Verification items for the finished model (mm, model axes). A direction names the side the tool comes from. Give positions to 0.01 mm unless a question says otherwise; leave off trailing zeros. Loops run counter-clockwise (first coordinate to the right, second up) from the corner with the lowest first, then second, coordinate; pieces in that order, holes last. Notation, with made-up numbers: (88.5, 40) - (102.5, 40) arc R26 cw to (102.5, 77) - close; hole circle Ø8 at (87, 27). An arc over 180 degrees is marked (long way). Answer in a Markdown table with one row per item.
```python
from build123d import *

# Parameters (mm, degrees)
F0_W     = 254
F0_H     = 76.2
F1_DEPTH = 6.35
F2_W     = 6.35
F2_H     = 6.35
F2_H_2   = 12.7
F2_H_3   = 31.75
F3_DEPTH = 6.35
F4_W     = 30.48
F4_H     = 6.35
F5_DEPTH = 6.351
F6_W     = 6.35
F6_H     = 12.7
F7_DEPTH = 6.351


with BuildPart() as f1:
    # F0 (on Front) → F1 (new body)
    with BuildSketch(Plane.XZ):
        with Locations((127, 38.1)):
            Rectangle(F0_W, F0_H)
    extrude(amount=F1_DEPTH)

    # F2 (on face) → F3 (cut, through all)
    with BuildSketch(Plane.XZ.offset(6.35)):
        with Locations((3.175, 3.175)):
            Rectangle(F2_W, F2_H)
        with Locations((3.175, 69.85)):
            Rectangle(F2_W, F2_H_2)
        with Locations((3.175, 34.925)):
            Rectangle(F2_W, F2_H_3)
        with Locations((250.825, 3.175)):
            Rectangle(F2_W, F2_H)
        with Locations((250.825, 34.925)):
            Rectangle(F2_W, F2_H_3)
        with Locations((250.825, 69.85)):
            Rectangle(F2_W, F2_H_2)
    extrude(amount=-F3_DEPTH, mode=Mode.SUBTRACT)

    # F4 (on face) → F5 (cut, through all)
    with BuildSketch(Plane.XZ.offset(6.35)):
        with Locations((15.24, 3.175)):
            Rectangle(F4_W, F4_H)
        with Locations((71.12, 3.175)):
            Rectangle(F4_W, F4_H)
        with Locations((127, 3.175)):
            Rectangle(F4_W, F4_H)
        with Locations((182.88, 3.175)):
            Rectangle(F4_W, F4_H)
        with Locations((238.76, 3.175)):
            Rectangle(F4_W, F4_H)
    extrude(amount=-F5_DEPTH, mode=Mode.SUBTRACT)

    # F6 (on face) → F7 (cut, through all)
    with BuildSketch(Plane.XZ.offset(6.35)):
        with Locations((85.725, 12.7)):
            Rectangle(F6_W, F6_H)
        with Locations((85.725, 57.15)):
            Rectangle(F6_W, F6_H)
        with Locations((168.275, 57.15)):
            Rectangle(F6_W, F6_H)
        with Locations((168.275, 12.7)):
            Rectangle(F6_W, F6_H)
    extrude(amount=-F7_DEPTH, mode=Mode.SUBTRACT)


solid = f1.part
```
Q1. Tool access check on faces 4 (the face through (251, -3, 63.5)), 5 (the face through (86, -3, 19.05)), 6 (the face through (239, -3, 6.35)), 7 (the face through (82.55, -3, 13)). Record the directions out of +Z, -Z, +X, -X, +Y, -Y that give a thin tool (end or side, any length) a straight path to the whole face; none if there is none.
Completed:
| item | result |
|---|---|
| face 4 | +Z, +X, +Y, -Y |
| face 5 | +Y, -Y |
| face 6 | -Z, +X, +Y, -Y |
| face 7 | -Z, +Y, -Y |
Q2. Draft check along X on faces 1 (the face through (168, -3, 50.8)), 2 (the face through (251, -3, 19.05)), 3 (the face through (254, -3, 57)). Enter one of: +X half, -X half, draft (parallel to the pull), parting line (faces both ways), or undercut.
Completed:
| item | result |
|---|---|
| face 1 | undercut |
| face 2 | draft |
| face 3 | +X half |
Q3. Sectioned sample at A-A (x = 135). Record the cut outline in (y, z), and give its area (3 significant figures).
Completed:
| item | result |
|---|---|
| outline | (-6.35, 6.35) - (0, 6.35) - (0, 76.2) - (-6.35, 76.2) - close |
| area | 444 mm^2 |
Q4. Sectioned sample at C-C (z = 40). Record the cut outline in (x, y).
Completed:
| item | result |
|---|---|
| outline | (6.35, -6.35) - (247.65, -6.35) - (247.65, 0) - (6.35, 0) - close |
Q5. Sectioned sample at B-B (y = -2.75). Give the number of separate pieces and of enclosed holes in the cut face, and give its area (3 significant figures).
Completed:
| item | result |
|---|---|
| separate pieces | 1 |
| enclosed holes | 2 |
| area | 17,500 mm^2 |
Q6. Go/stop test with flat-tipped pins: P1, Ø3, axis at x = 4, y = -2, coming from the -Z side; P2, Ø2, axis at y = -4.5, z = 22, coming from the -X side; P3, Ø1.9, axis at y = -2.5, z = 4.5, coming from the +X side. Record where each tip stops, or that it passes through.
Completed:
| item | result |
|---|---|
| P1 | z = 6.35 |
| P2 | x = 6.35 |
| P3 | x = 223.52 |
Q7. Thickness scan on line 1 (X direction, y = -4.75, z = 60); line 2 (X direction, y = -6, z = 26.5); line 3 (Z direction, x = 65, y = -4). Record the ranges inside material, lowest first.
Completed:
| item | result |
|---|---|
| line 1 | 0 to 82.55, 88.9 to 165.1, 171.45 to 254 |
| line 2 | 6.35 to 247.65 |
| line 3 | 6.35 to 76.2 |
